Design review of the part built by this model. Coordinates are the model's own, in mm. Coordinates: 2 decimals unless noted, no trailing zeros. Loops run counter-clockwise (first coordinate to the right, second up) from the corner with the lowest first, then second, coordinate; pieces in that order, holes last.
Q1. Wall thickness on probe 1 along Y at (x, z) = (22.1, 4.5); probe 2 along Y at (x, z) = (30, 3); probe 3 along Z at (x, y) = (26.5, 17.5): over which ranges is each line inside the solid? List them lowest first.
Q2. For P1, Ø5.5, axis at x = 16.5, y = 5.5, coming from the +Z side; P2, Ø2, axis at x = 15, y = 5.5, coming from the -Z side; P3, Ø3.5, axis at x = 26, y = 15, coming from the +Z side, all flat-tipped, find the tip position at first contact; note any pin that passes through.
Q3. Add section A-A on x = 18. Give the boundary of the cut face in (y, z), and give its area (3 significant figures).
Q4. Add section B-B on y = 14.25. Give the boundary of the cut face in (x, z), and give its area (3 significant figures).
```python
from build123d import *

# Parameters (mm, degrees)
SKETCH1_W                = 44.2
SKETCH1_H                = 20
BOSS_EXTRUDE1_DEPTH      = 50.8
SKETCH2_R                = 0.863384433
CUT_EXTRUDE1_DEPTH       = 6.35
CHAMFER1_SIZE            = 0.508
CHAMFER1_OF_MIRROR2_SIZE = 0.508


with BuildPart() as part:
    # Sketch1 → Boss-Extrude1 (new body)
    with BuildSketch(Plane.XY):
        with Locations((22.1, 10)):
            Rectangle(SKETCH1_W, SKETCH1_H)
    extrude(amount=BOSS_EXTRUDE1_DEPTH)

    # Sketch2 → Cut-Extrude1 (cut)
    with BuildSketch(Plane(origin=(0, 0, 0), x_dir=(-1, 0, 0), z_dir=(0, 0, -1))):
        with Locations((-22.1, 10)):
            Circle(SKETCH2_R)
        Polygon((-25.088596798, 18.34725), (-29.011403202, 18.34725), (-30.972806404, 14.95), (-29.011403202, 11.55275), (-25.088596798, 11.55275), (-23.127193596, 14.95), align=None)
        Polygon((-15.188596798, 18.34725), (-19.111403202, 18.34725), (-21.072806404, 14.95), (-19.111403202, 11.55275), (-15.188596798, 11.55275), (-13.227193596, 14.95), align=None)
        Polygon((-15.188596798, 8.44725), (-19.111403202, 8.44725), (-21.072806404, 5.05), (-19.111403202, 1.65275), (-15.188596798, 1.65275), (-13.227193596, 5.05), align=None)
        Polygon((-25.088596798, 8.44725), (-29.011403202, 8.44725), (-30.972806404, 5.05), (-29.011403202, 1.65275), (-25.088596798, 1.65275), (-23.127193596, 5.05), align=None)
    cut_extrude1 = extrude(amount=-CUT_EXTRUDE1_DEPTH, mode=Mode.SUBTRACT)

    # Chamfer1
    chamfer1_edges = [part.edges().sort_by_distance(p)[0] for p in [
        (24.107895197, 6.748625, 0),
        (27.05, 8.44725, 0),
        (29.992104803, 6.748625, 0),
        (29.992104803, 3.351375, 0),
        (27.05, 1.65275, 0),
        (24.107895197, 3.351375, 0),
        (14.207895197, 6.748625, 0),
        (17.15, 8.44725, 0),
        (20.092104803, 6.748625, 0),
        (20.092104803, 3.351375, 0),
        (17.15, 1.65275, 0),
        (14.207895197, 3.351375, 0),
        (14.207895197, 16.648625, 0),
        (17.15, 18.34725, 0),
        (20.092104803, 16.648625, 0),
        (20.092104803, 13.251375, 0),
        (17.15, 11.55275, 0),
        (14.207895197, 13.251375, 0),
        (24.107895197, 16.648625, 0),
        (27.05, 18.34725, 0),
        (29.992104803, 16.648625, 0),
        (29.992104803, 13.251375, 0),
        (27.05, 11.55275, 0),
        (24.107895197, 13.251375, 0),
    ]]
    chamfer(chamfer1_edges, length=CHAMFER1_SIZE)

    # Mirror2: Cut-Extrude1 across plane
    add(cut_extrude1.mirror(Plane(origin=(0, 0, 25.4), x_dir=(1, 0, 0), z_dir=(0, 0, -1))), mode=Mode.SUBTRACT)

    # Chamfer1 of Mirror2
    chamfer1_of_mirror2_edges = [part.edges().sort_by_distance(p)[0] for p in [
        (24.107895197, 6.748625, 50.8),
        (27.05, 8.44725, 50.8),
        (29.992104803, 6.748625, 50.8),
        (29.992104803, 3.351375, 50.8),
        (27.05, 1.65275, 50.8),
        (24.107895197, 3.351375, 50.8),
        (14.207895197, 6.748625, 50.8),
        (17.15, 8.44725, 50.8),
        (20.092104803, 6.748625, 50.8),
        (20.092104803, 3.351375, 50.8),
        (17.15, 1.65275, 50.8),
        (14.207895197, 3.351375, 50.8),
        (14.207895197, 16.648625, 50.8),
        (17.15, 18.34725, 50.8),
        (20.092104803, 16.648625, 50.8),
        (20.092104803, 13.251375, 50.8),
        (17.15, 11.55275, 50.8),
        (14.207895197, 13.251375, 50.8),
        (24.107895197, 16.648625, 50.8),
        (27.05, 18.34725, 50.8),
        (29.992104803, 16.648625, 50.8),
        (29.992104803, 13.251375, 50.8),
        (27.05, 11.55275, 50.8),
        (24.107895197, 13.251375, 50.8),
    ]]
    chamfer(chamfer1_of_mirror2_edges, length=CHAMFER1_OF_MIRROR2_SIZE)


solid = part.part
```
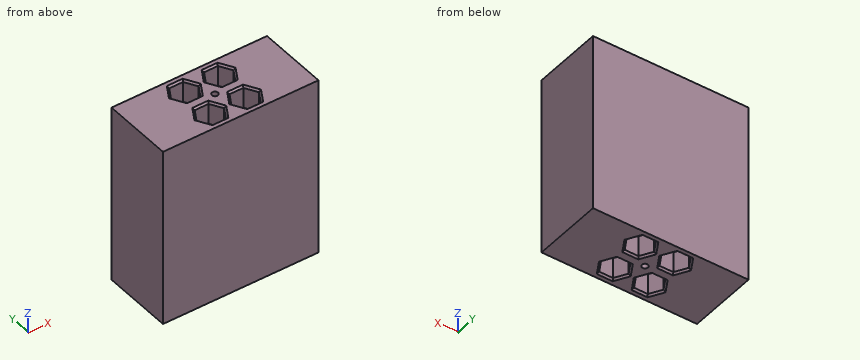
Entries:
1. probe 1: y = 0 to 9.14, 10.86 to 20
1. probe 2: y = 0 to 3.37, 6.73 to 13.27, 16.63 to 20
1. probe 3: z = 6.35 to 44.45
2. P1: stops at z = 50.43
2. P2: stops at z = 6.35
2. P3: stops at z = 44.45
3. outline: (0, 0) - (1.14, 0) - (1.65, 0.51) - (1.65, 6.35) - (8.45, 6.35) - (8.45, 0.51) - (8.96, 0) - (11.04, 0) - (11.55, 0.51) - (11.55, 6.35) - (18.35, 6.35) - (18.35, 0.51) - (18.86, 0) - (20, 0) - (20, 50.8) - (18.86, 50.8) - (18.35, 50.29) - (18.35, 44.45) - (11.55, 44.45) - (11.55, 50.29) - (11.04, 50.8) - (8.96, 50.8) - (8.45, 50.29) - (8.45, 44.45) - (1.65, 44.45) - (1.65, 50.29) - (1.14, 50.8) - (0, 50.8) - close
3. area: 842 mm2
4. outline: (0, 0) - (13.04, 0) - (13.63, 0.51) - (13.63, 6.35) - (20.67, 6.35) - (20.67, 0.51) - (21.26, 0) - (22.94, 0) - (23.53, 0.51) - (23.53, 6.35) - (30.57, 6.35) - (30.57, 0.51) - (31.16, 0) - (44.2, 0) - (44.2, 50.8) - (31.16, 50.8) - (30.57, 50.29) - (30.57, 44.45) - (23.53, 44.45) - (23.53, 50.29) - (22.94, 50.8) - (21.26, 50.8) - (20.67, 50.29) - (20.67, 44.45) - (13.63, 44.45) - (13.63, 50.29) - (13.04, 50.8) - (0, 50.8) - close
4. area: 2,070 mm2
